Autodesk Inventor part; units mm, degrees
ref_plane "YZ Plane" through (0, 0, 0) normal (1, 0, 0) x (0, 1, 0)
ref_plane "XZ Plane" through (0, 0, 0) normal (0, 1, 0) x (-1, 0, 0)
ref_plane "XY Plane" through (0, 0, 0) normal (0, 0, 1) x (1, 0, 0)
sketch "Block1" plane through (0, 0, 0) normal (0, 0, 1) x (1, 0, 0)
  line L0 (-17.5911, -8.406) -> (-17.5911, -2.6569)
  arc A0 (-15.6308, 0.6431) -> (-17.4939, -2.2845) centre (9.5285, -17.4245) ccw
  arc A1 (-17.4939, -2.2845) -> (-17.5911, -2.6569) centre (-16.8291, -2.6569) ccw
  line L1 (-13.0521, -3.6322) -> (-2.9855, -3.6322)
  line L2 (-2.9855, -3.6322) -> (-2.9855, -10.0136)
  line L3 (-2.9855, -10.0136) -> (-13.0521, -10.0136)
  line L4 (-13.0521, -10.0136) -> (-13.0521, -3.6322)
  ellipse E0 centre (-8.0188, -3.6322) end of major axis (-8.0188, -7.4704) minor radius 2.9685
  point P0 (-13.9703, -5.5207)
  point P1 (-17.5911, -2.4593)
  dimension "d111" = 0.762
sketch "Block2" plane through (0, 0, 0) normal (0, 0, 1) x (1, 0, 0)
  line L0 (-7.8958, -2.4967) -> (-7.8958, -8.4058)
  line L1 (-8.6339, -9.168) -> (-16.8291, -9.168)
  ellipse E0 centre (-12.6564, -2.1178) end of major axis (-12.6564, -6.4967) minor radius 3.853 (-9.6585, 0.6329) -> (-15.6415, 0.6509) ccw
  arc A0 (-7.8958, -2.4967) -> (-9.6091, 0.6391) centre (-35.8892, -15.7554) ccw
  line L2 (-17.6018, -8.3981) -> (-17.6018, -2.6491)
  arc A1 (-15.6415, 0.6509) -> (-17.5045, -2.2766) centre (9.5178, -17.4167) ccw
  arc A2 (-17.5045, -2.2766) -> (-17.6018, -2.6491) centre (-16.8398, -2.6491) ccw
  line L3 (-13.0627, -3.6243) -> (-2.9962, -3.6243)
  line L4 (-2.9962, -3.6243) -> (-2.9962, -10.0058)
  line L5 (-2.9962, -10.0058) -> (-13.0627, -10.0058)
  line L6 (-13.0627, -10.0058) -> (-13.0627, -3.6243)
  ellipse E1 centre (-8.0295, -3.6243) end of major axis (-8.0295, -7.4625) minor radius 2.9685
  point P0 (-12.2397, -5.1213)
sketch "Block3" plane through (0, 0, 0) normal (0, 0, 1) x (1, 0, 0)
  arc A0 (-17.5911, -8.406) -> (-16.8291, -9.168) centre (-16.8291, -8.406) ccw
  arc A1 (-8.6339, -9.168) -> (-7.8719, -8.406) centre (-8.6339, -8.406) ccw
  line L0 (-7.8958, -2.4967) -> (-7.8958, -8.4058)
  line L1 (-8.6339, -9.168) -> (-16.8291, -9.168)
  ellipse E0 centre (-12.6564, -2.1178) end of major axis (-12.6564, -6.4967) minor radius 3.853 (-9.6585, 0.6329) -> (-15.6415, 0.6509) ccw
  arc A2 (-7.8958, -2.4967) -> (-9.6091, 0.6391) centre (-35.8892, -15.7554) ccw
  line L2 (-17.6018, -8.3981) -> (-17.6018, -2.6491)
  arc A3 (-15.6415, 0.6509) -> (-17.5045, -2.2766) centre (9.5178, -17.4167) ccw
  arc A4 (-17.5045, -2.2766) -> (-17.6018, -2.6491) centre (-16.8398, -2.6491) ccw
  line L3 (-13.0627, -3.6243) -> (-2.9962, -3.6243)
  line L4 (-2.9962, -3.6243) -> (-2.9962, -10.0058)
  line L5 (-2.9962, -10.0058) -> (-13.0627, -10.0058)
  line L6 (-13.0627, -10.0058) -> (-13.0627, -3.6243)
  ellipse E1 centre (-8.0295, -3.6243) end of major axis (-8.0295, -7.4625) minor radius 2.9685
  point P0 (-12.6868, -8.3844)
  dimension "d110" = 0.762
sketch "Block4" plane through (0, 0, 0) normal (0, 0, 1) x (1, 0, 0)
  arc A0 (-17.5911, -8.406) -> (-16.8291, -9.168) centre (-16.8291, -8.406) ccw
  arc A1 (-8.6339, -9.168) -> (-7.8719, -8.406) centre (-8.6339, -8.406) ccw
  line L0 (-7.8958, -2.4967) -> (-7.8958, -8.4058)
  line L1 (-8.6339, -9.168) -> (-16.8291, -9.168)
  ellipse E0 centre (-12.6564, -2.1178) end of major axis (-12.6564, -6.4967) minor radius 3.853 (-9.6585, 0.6329) -> (-15.6415, 0.6509) ccw
  arc A2 (-7.8958, -2.4967) -> (-9.6091, 0.6391) centre (-35.8892, -15.7554) ccw
  line L2 (-17.6018, -8.3981) -> (-17.6018, -2.6491)
  arc A3 (-15.6415, 0.6509) -> (-17.5045, -2.2766) centre (9.5178, -17.4167) ccw
  arc A4 (-17.5045, -2.2766) -> (-17.6018, -2.6491) centre (-16.8398, -2.6491) ccw
  line L3 (-13.0627, -3.6243) -> (-2.9962, -3.6243)
  line L4 (-2.9962, -3.6243) -> (-2.9962, -10.0058)
  line L5 (-2.9962, -10.0058) -> (-13.0627, -10.0058)
  line L6 (-13.0627, -10.0058) -> (-13.0627, -3.6243)
  ellipse E1 centre (-8.0295, -3.6243) end of major axis (-8.0295, -7.4625) minor radius 2.9685
  point P0 (-12.6868, -8.3844)
sketch "Block5" plane through (0, 0, 0) normal (0, 0, 1) x (1, 0, 0)
  ellipse E0 centre (-12.7876, -1.8459) end of major axis (-12.7876, -5.6516) minor radius 3.3457 (-10.6846, 1.114) -> (-14.8941, 1.1109) ccw
  arc A0 (-15.6984, 0.3796) -> (-14.8859, 1.1184) centre (-85.8065, 78.298) ccw
  arc A1 (-10.6894, 1.1184) -> (-9.8669, 0.3716) centre (60.1779, 78.3469) ccw
  point P0 (-12.7899, 8.9309)
sketch "Block6" plane through (0, 0, 0) normal (0, 0, 1) x (1, 0, 0)
  arc A0 (-10.9697, 1.4333) -> (-15.1792, 1.1122) centre (-12.8849, -1.2117) ccw
  line L0 (-15.1792, 1.1122) -> (-17.7718, -1.4473)
  line L1 (-10.8839, 1.361) -> (-8.0119, -1.4473)
  line L2 (-17.7718, -1.4473) -> (-8.0119, -1.4473)
  arc A1 (-10.8839, 1.361) -> (-10.9697, 1.4333) centre (-11.4166, 0.8161) ccw
  point P0 (-12.0633, -0.3449)
  point P1 (-10.9214, 1.3977)
  dimension "d153" = 0.762
sketch "Sketch1" plane through (0, 0, 0) normal (0, 0, 1) x (1, 0, 0)
  line L0 (-19.9256, -1.4064) -> (-6.1106, -1.4064)
  line L1 (-6.1106, -1.4064) -> (-6.1106, -8.6156)
  line L2 (-6.1106, -8.6156) -> (-19.9256, -8.6156)
  line L3 (-19.9256, -8.6156) -> (-19.9256, -1.4064)
extrude "Extrusion1" add sketch "Sketch1" along normal blind 1.524
sketch "Sketch13" plane through (0, 0, 1.524) normal (0, 0, 1) x (1, 0, 0)
  arc A0 (-10.8192, 2.023) -> (-15.0287, 1.7019) centre (-12.7344, -0.622) ccw
  line L0 (-15.0287, 1.7019) -> (-17.6213, -0.8576)
  line L1 (-10.7334, 1.9507) -> (-7.8614, -0.8576)
  line L2 (-17.6213, -0.8576) -> (-7.8614, -0.8576)
  arc A1 (-10.7334, 1.9507) -> (-10.8192, 2.023) centre (-11.2661, 1.4058) ccw
  point P0 (0, 0)
  point P1 (0, 0)
  point P2 (0, 0)
extrude "Extrusion8" add sketch "Sketch13" against normal blind 1.524
sketch "Sketch16" plane through (0, 0, 1.524) normal (0, 0, 1) x (1, 0, 0)
  line L0 (-19.2542, -0.6452) -> (-6.1548, -0.6452)
  line L1 (-5.3928, -1.4072) -> (-5.3928, -8.5513)
  line L2 (-6.1548, -9.3133) -> (-19.2542, -9.3133)
  line L3 (-20.0162, -8.5513) -> (-20.0162, -1.4072)
  arc A0 (-19.2542, -0.6452) -> (-20.0162, -1.4072) centre (-19.2542, -1.4072) ccw
  arc A1 (-20.0162, -8.5513) -> (-19.2542, -9.3133) centre (-19.2542, -8.5513) ccw
  arc A2 (-6.1548, -9.3133) -> (-5.3928, -8.5513) centre (-6.1548, -8.5513) ccw
  arc A3 (-5.3928, -1.4072) -> (-6.1548, -0.6452) centre (-6.1548, -1.4072) ccw
  point P0 (0, 0)
  dimension "d177" = 0.762
  dimension "d178" = 0.762
  dimension "d179" = 0.762
  dimension "d180" = 0.762
extrude "Extrusion9" add sketch "Sketch16" against normal blind 1.524
hole "Hole9" at (-19.2355, -4.93, 1.524) direction (0, 0, -1) diameter 1.016 depth 1.524
hole "Hole10" at (-6.1975, -4.9172, 1.524) direction (0, 0, -1) diameter 1.016 depth 1.524
properties part number "headplateLP_protector"
Can you work these out from the model? Positions are in its coordinate system, mm. A direction names the side the tool comes from. Round coordinates to 2 decimals unless told otherwise and drop trailing zeros. Loops run counter-clockwise (first coordinate to the right, second up) from the corner with the lowest first, then second, coordinate; pieces in that order, holes last. Notation, with made-up numbers: M -24.75,83 L 33.25,83 A23 cw 33.25,105 Z; hole C -36.5,60.25 d8. An arc over 180 degrees is marked long. Write item = value, one per line. Start each with the question number.
(1) Which directions (+Z, -Z, +X, -X, +Y, -Y) give clear straight access to the entire face, cutting with the end or side of a thin tool? Please do faces 4 (the face through (-19.74, -4.86, 0.75)), 5 (the face through (-7, -0.645, 1)), 6 (the face through (-18, -0.645, 1)).
(2) Suppose I cut it at B-B on x = -6.5. Write out the boundary of the cut face in (y, z), plus the area to 3 significant figures.
(3) If we mould it in two halves opening along Y, with no side actions, what happens to faces 1 (the face through (-6.35, -5.4, 0.75)), 2 (the face through (-20.016, -5, 1)), 3 (the face through (-13, -9.313, 1))? For each: released by +Y, released by -Y, zero draft, split by the parting line, or undercut.
(4) I'm going to push flat-ended pins straight in: P1, Ø0.8, axis at x = -6.2, y = -4.92, coming from the -Z side; P2, Ø0.5, axis at x = -18, z = 0.5, coming from the +Y side. Where does each tip first touch, or does it pass through?
(5) Suppose I cut it at A-A on y = -4.93. Write out the boundary of the cut face in (x, z).
(6) Suppose I cut it at D-D on y = -1. Write out the boundary of the cut face in (x, z).
(7) Suppose I cut it at C-C on z = 1.1. Write out the boundary of the cut face in (x, y).
(8) I need wall thicknesses on line 1 along X through (y, z) = (-4.93, 1); line 2 along Y through (x, z) = (-18.25, 0.3); line 3 along X through (y, z) = (-5.25, 0.85). Which ranges of each line are inside material? Lowest first, please.
Answer block:
q1.face_4 = +Z, -Z
q1.face_5 = +Z, -Z, +X, +Y
q1.face_6 = +Z, -Z, -X, +Y
q2.outline = M -9.31,0 L -5.33,0 L -5.33,1.52 L -9.31,1.52 Z; M -4.51,0 L -0.65,0 L -0.65,1.52 L -4.51,1.52 Z
q2.area = 12.0 mm²
q3.face_1 = undercut
q3.face_2 = zero draft
q3.face_3 = released by -Y
q4.P1 = through
q4.P2 = -0.65
q5.outline = M -20.02,0 L -19.74,0 L -19.74,1.52 L -20.02,1.52 Z; M -18.73,0 L -6.71,0 L -6.71,1.52 L -18.73,1.52 Z; M -5.69,0 L -5.39,0 L -5.39,1.52 L -5.69,1.52 Z
q6.outline = M -19.9,0 L -5.51,0 L -5.51,1.52 L -19.9,1.52 Z
q7.outline = M -20.02,-8.55 A0.76 ccw -19.25,-9.31 L -6.15,-9.31 A0.76 ccw -5.39,-8.55 L -5.39,-1.41 A0.76 ccw -6.15,-0.65 L -8.08,-0.65 L -10.73,1.95 A0.76 ccw -10.82,2.02 A3.27 ccw -15.03,1.7 L -17.41,-0.65 L -19.25,-0.65 A0.76 ccw -20.02,-1.41 Z; hole C -19.24,-4.93 d1.02; hole C -6.2,-4.92 d1.02
q8.line_1 = -20.02 to -19.74, -18.73 to -6.71, -5.69 to -5.39
q8.line_2 = -9.31 to -0.65
q8.line_3 = -20.02 to -19.63, -18.84 to -6.58, -5.81 to -5.39
